The listing builds one solid part. Answer for the finished solid, in the listing's coordinates (mm). Round coordinates to 2 decimals unless told otherwise and drop trailing zeros. Write each loop counter-clockwise with the first axis right and the second up, starting at its lowest first coordinate (ties: lowest second). Pieces come first, ordered by that corner, then holes. Notation, with made-up numbers: (67.25, 41) - (125.25, 41) arc R30 cw to (125.25, 78) - close; hole circle Ø4 at (24, -17.5). An arc over 180 degrees is marked (long way). Return JSON: item names as keys, results as strings. Group by question number.
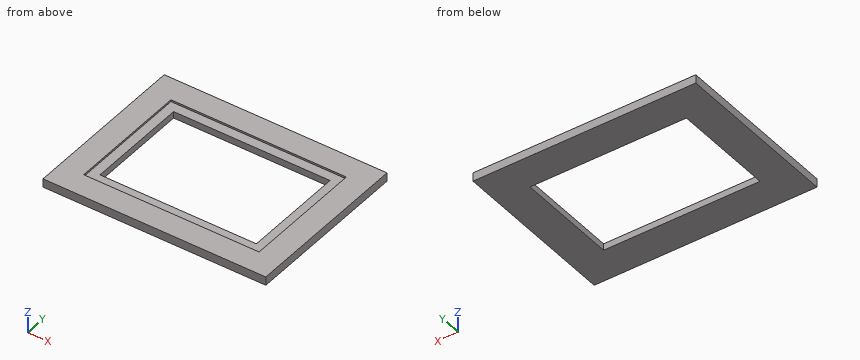
from build123d import *

# Parameters (mm, degrees)
SKETCH1_W           = 470
SKETCH1_H           = 357
BOSS_EXTRUDE1_DEPTH = 18
SKETCH3_W           = 370
SKETCH3_H           = 257
CUT_EXTRUDE1_DEPTH  = 4
SKETCH4_W           = 330
SKETCH4_H           = 217
CUT_EXTRUDE2_DEPTH  = 591.376998197


with BuildPart() as part:
    # Sketch1 → Boss-Extrude1 (new body)
    with BuildSketch(Plane.XY):
        with Locations((235, 178.5)):
            Rectangle(SKETCH1_W, SKETCH1_H)
    extrude(amount=BOSS_EXTRUDE1_DEPTH)

    # Sketch3 → Cut-Extrude1 (cut)
    with BuildSketch(Plane.XY.offset(18)):
        with Locations((235, 178.5)):
            Rectangle(SKETCH3_W, SKETCH3_H)
    extrude(amount=-CUT_EXTRUDE1_DEPTH, mode=Mode.SUBTRACT)

    # Sketch4 → Cut-Extrude2 (cut, through all)
    with BuildSketch(Plane.XY.offset(14)):
        with Locations((235, 178.5)):
            Rectangle(SKETCH4_W, SKETCH4_H)
    extrude(amount=-CUT_EXTRUDE2_DEPTH, mode=Mode.SUBTRACT)


solid = part.part
(1) Find section A-A (x = 154.5). Write down the section's boundary in (y, z), plus the area to 3 significant figures.
(2) Find section B-B (y = 112). Write down the section's boundary in (x, z).
(3) Consider line 1 (X direction, y = 201.5, z = 10); line 2 (Y direction, x = 102, z = 7.75); line 3 (Y direction, x = 274, z = 16). Determine where each line is inside the solid, lowest interval first.
(4) Find section C-C (z = 5.25). Write down the section's boundary in (x, y).
Check sheet entries:
{
 "1": {"outline": "(0, 0) - (70, 0) - (70, 14) - (50, 14) - (50, 18) - (0, 18) - close; (287, 0) - (357, 0) - (357, 18) - (307, 18) - (307, 14) - (287, 14) - close", "area": "2,360 mm^2"},
 "2": {"outline": "(0, 0) - (70, 0) - (70, 14) - (50, 14) - (50, 18) - (0, 18) - close; (400, 0) - (470, 0) - (470, 18) - (420, 18) - (420, 14) - (400, 14) - close"},
 "3": {"line 1": "x = 0 to 70, 400 to 470", "line 2": "y = 0 to 70, 287 to 357", "line 3": "y = 0 to 50, 307 to 357"},
 "4": {"outline": "(0, 0) - (470, 0) - (470, 357) - (0, 357) - close; hole (70, 70) - (400, 70) - (400, 287) - (70, 287) - close"}
}
